Job drawing, mm, ordinate dimensions from the low corner. One solid piece. A direction names the side the tool comes from. Give positions to 0.01 mm unless a question says otherwise; leave off trailing zeros. Write each loop counter-clockwise with the first axis right and the second up, starting at its lowest first coordinate (ties: lowest second). Pieces come first, ordered by that corner, then holes. Notation, with made-up numbers: M 62,56 L 119,56 A21 cw 119,71 Z; hole C 21.5,-24 d11. An arc over 180 degrees is marked long. Use CSV: the item, a comma, the result in double quotes. Start each with the question number.
Item 1: Cut at A-A (y = 53). List the corners of the cut face in (x, z).
Item 2: Cut at C-C (x = 26). List the corners of the cut face in (y, z).
Item 3: Which spindle directions (+Z, -Z, +X, -X, +Y, -Y) get a long thin tool onto all of the face, cutting with end or side? Do the marked faces 1, 2, 3 and 4. Say none if no direction does.
Item 4: Pin check, flat tips, straight feed: pin 1 (9.5 mm diameter, centred on y = 17.5, z = 13.5, fed in from +X); pin 2 (6 mm diameter, centred on x = 18.5, y = 42.5, fed in from +Z); pin 3 (2 mm diameter, centred on x = 9.5, z = 26.5, fed in from +Y). Stop position of each tip, or through.
Item 5: Cut at D-D (y = 24). List the corners of the cut face in (x, z), then the cut area to 3 significant figures.
Item 6: Mould opens along X. For the marked faces 5 and 6 say: released by +X, released by -X, zero draft, split by the parting line, or undercut.
Item 7: Drill centre lines: line 1 (Z direction, x = 42, y = 2.2); line 2 (X direction, y = 1, z = 16); line 3 (Z direction, x = 7, y = 19). Where is each one in solid material? Low to high. Write a range as [from, to].
Item 8: Cut at B-B (z = 16). Count the separate pieces of the cut face and the enclosed holes in it, then the cut area to 3 significant figures.
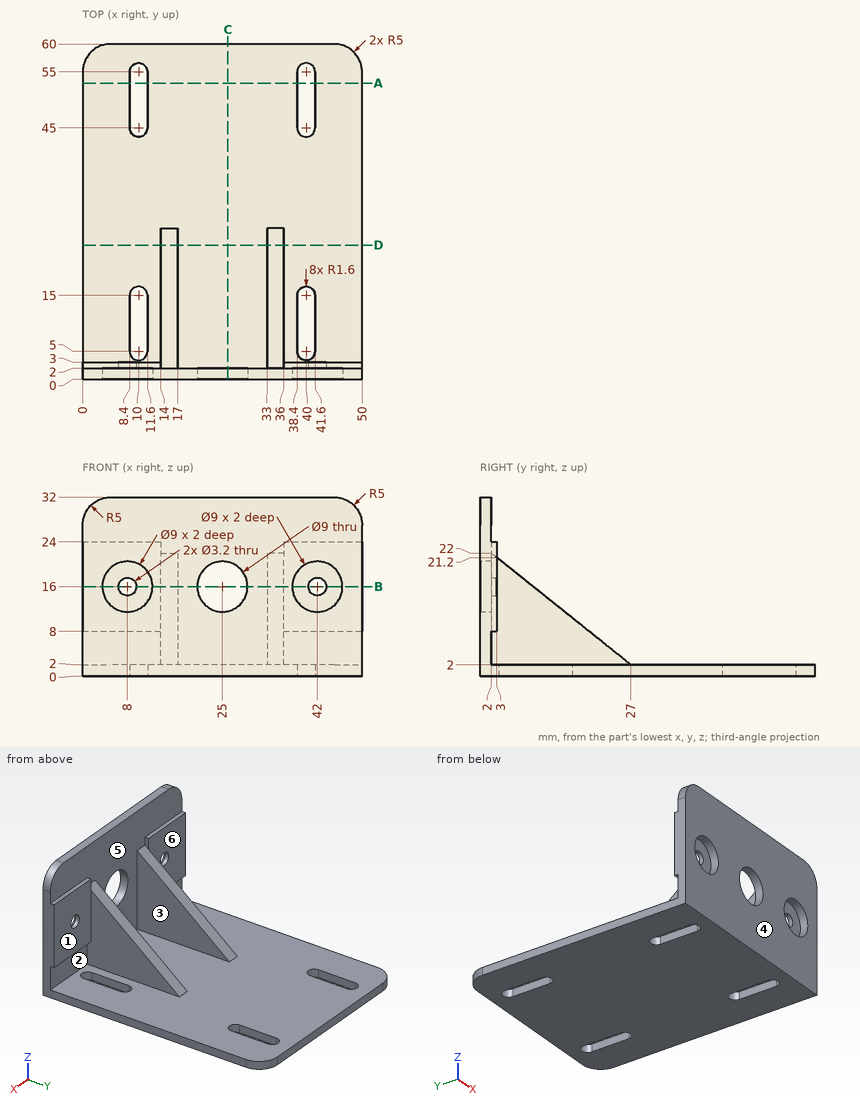
Worked answers:
1,outline,"M 0,0 L 8.4,0 L 8.4,2 L 0,2 Z; M 11.6,0 L 38.4,0 L 38.4,2 L 11.6,2 Z; M 41.6,0 L 50,0 L 50,2 L 41.6,2 Z"
2,outline,"M 0,0 L 60,0 L 60,2 L 2,2 L 2,11.61 L 0,11.61 Z; M 0,20.39 L 2,20.39 L 2,32 L 0,32 Z"
3,face 1,"+Z, +X, +Y"
3,face 2,"+X, +Y"
3,face 3,"+Z, +Y"
3,face 4,"+Z, -Z, +X, -X, -Y"
4,pin 1,"stops at x = 36"
4,pin 2,"stops at z = 2"
4,pin 3,"stops at y = 2"
5,outline,"M 0,0 L 50,0 L 50,2 L 36,2 L 36,4.4 L 33,4.4 L 33,2 L 17,2 L 17,4.4 L 14,4.4 L 14,2 L 0,2 Z"
5,area,"114 mm^2"
6,face 5,"undercut"
6,face 6,"zero draft"
7,line 1,"z = [0, 2], [8, 14.4], [17.6, 24]"
7,line 2,"x = [0, 3.5], [12.5, 20.5], [29.5, 37.5], [46.5, 50]"
7,line 3,"z = [0, 2]"
8,separate pieces,"4"
8,enclosed holes,"0"
8,area,"113 mm^2"
